from build123d import *

# Parameters (mm, degrees)
F1_DEPTH = 25.4
F2_R     = 6.35
F3_DEPTH = 12.7
F5_DEPTH = 25.4
F7_DEPTH = 12.7
F9_DEPTH = 12.7


with BuildPart() as f1:
    # F0 (on Front) → F1 (new body)
    with BuildSketch(Plane.XZ):
        Polygon((-56.1258053064, 50.8), (-68.8258053064, 50.8), (-68.8258053064, 0), (-11.6758053064, 0), (-11.6758053064, 12.7), (-56.1258053064, 12.7), align=None)
    extrude(amount=F1_DEPTH)

    # F2 (on face) → F3 (cut)
    with BuildSketch(Plane.XY.offset(12.7)):
        with Locations((-43.4258053064, -12.7)):
            Circle(F2_R)
        with Locations((-24.3758053064, -12.7)):
            Circle(F2_R)
    extrude(amount=-F3_DEPTH, mode=Mode.SUBTRACT)

    # F4 (on face) → F5 (cut)
    with BuildSketch(Plane.XY.offset(12.7)):
        with BuildLine():
            ThreePointArc((-24.3758053064, 0), (-15.3955491853, -3.7197438789), (-11.6758053064, -12.7))
            Line((-11.6758053064, -12.7), (-11.6758053064, 0))
            Line((-11.6758053064, 0), (-24.3758053064, 0))
        make_face()
        with BuildLine():
            Line((-11.6758053064, -25.4), (-11.6758053064, -12.7))
            ThreePointArc((-11.6758053064, -12.7), (-15.3955491853, -21.6802561211), (-24.3758053064, -25.4))
            Line((-24.3758053064, -25.4), (-11.6758053064, -25.4))
        make_face()
    extrude(amount=-F5_DEPTH, mode=Mode.SUBTRACT)

    # F6 (on face) → F7 (cut)
    with BuildSketch(Plane.YZ.offset(-56.1258053064)):
        with BuildLine():
            ThreePointArc((-19.040173462, 31.75), (-12.690173462, 38.1), (-6.340173462, 31.75))
            Line((-6.340173462, 31.75), (-6.340173462, 50.8))
            Line((-6.340173462, 50.8), (-19.040173462, 50.8))
            Line((-19.040173462, 50.8), (-19.040173462, 31.75))
        make_face()
        with BuildLine():
            ThreePointArc((-19.040173462, 31.75), (-12.690173462, 25.4), (-6.340173462, 31.75))
            ThreePointArc((-6.340173462, 31.75), (-12.690173462, 38.1), (-19.040173462, 31.75))
        make_face()
    extrude(amount=-F7_DEPTH, mode=Mode.SUBTRACT)

    # F8 (on face) → F9 (cut)
    with BuildSketch(Plane.YZ.offset(-56.1258053064)):
        with BuildLine():
            ThreePointArc((-25.4, 44.5000978606), (-22.682681328, 47.7661903137), (-19.040173462, 49.9532699015))
            Line((-19.040173462, 49.9532699015), (-19.040173462, 50.8))
            Line((-19.040173462, 50.8), (-25.4, 50.8))
            Line((-25.4, 50.8), (-25.4, 44.5000978606))
        make_face()
        with BuildLine():
            Line((-6.340173462, 50.8), (-6.340173462, 50.3012942354))
            ThreePointArc((-6.340173462, 50.3012942354), (-2.7361670375, 48.2166562079), (0, 45.0785089908))
            Line((0, 45.0785089908), (0, 50.8))
            Line((0, 50.8), (-6.340173462, 50.8))
        make_face()
    extrude(amount=-F9_DEPTH, mode=Mode.SUBTRACT)


solid = f1.part
Could you check a few things on this model? Use its own coordinates, in mm. A direction names the side the tool comes from. Round coordinates to 2 decimals unless told otherwise and drop trailing zeros. Write each loop counter-clockwise with the first axis right and the second up, starting at its lowest first coordinate (ties: lowest second). Pieces come first, ordered by that corner, then holes. Notation, with made-up numbers: (11.5, -16) - (51.5, -16) arc R18 ccw to (51.5, 4) - close; hole circle Ø6 at (48, 72.25). An arc over 180 degrees is marked (long way). Put each result on its own line as item: value. Start each with the question number.
(1) I want a section at B-B, the plane x = -45.5. Please give me the cut outline in (y, z).
(2) I want a section at D-D, the plane x = -52.5. Please give me the cut outline in (y, z), plus the area to 3 significant figures.
(3) For faces 5 (the flat face through (-62, -6.34, 41)), 6 (the flat face through (-34, -13, 12.7)), 7 (the cylindrical face through (-62.387, -2.781, 48.254)), which set-ups out of +Z, -Z, +X, -X, +Y, -Y let a thin tool reach every point of the face, with its end or its side?
(4) Thinking about a two-plate mould opening in X: for faces 1 (the cylindrical face through (-48.465, -16.564, 6.439)), 2 (the cylindrical face through (-62.4, -12.8, 25.4)), 3 (the flat face through (-56.126, -13, 23)), 4 (the cylindrical face through (-29.415, -16.564, 6.439)), which applies, released by +X, released by -X, zero draft, split by the parting line, or undercut?
(5) I want a section at A-A, the plane z = 33.5. Please give me the cut outline in (x, y).
(6) I need wall thicknesses on probe 1 along Y at (x, z) = (-64, 35.5); probe 2 along Z at (x, y) = (-52, -6); probe 3 along Y at (x, z) = (-65.5, 29). Which ranges of each line are inside material? Lowest first, please.
(7) Will these pins go through, and if not, where does the flat tip stop? pin 1 (12 mm diameter, centred on x = -48.5, z = 29.5, fed in from -Y); pin 2 (12.5 mm diameter, centred on x = -23, y = -15, fed in from +Z).
(8) I want a section at C-C, the plane y = -13.5. Please give me the cut outline in (x, z), plus the area to 3 significant figures.
Here are the results:
1. outline: (-25.4, 0) - (-18.7, 0) - (-18.7, 12.7) - (-25.4, 12.7) - close; (-6.7, 0) - (0, 0) - (0, 12.7) - (-6.7, 12.7) - close
2. outline: (-25.4, 0) - (0, 0) - (0, 12.7) - (-25.4, 12.7) - close
2. area: 323 mm^2
3. face 5: +Z, +X, -X
3. face 6: +Z, +X, +Y, -Y
3. face 7: +Z, +X, -X, +Y
4. face 1: undercut
4. face 2: zero draft
4. face 3: released by +X
4. face 4: undercut
5. outline: (-68.83, -25.4) - (-56.13, -25.4) - (-56.13, -19.04) - (-68.83, -19.04) - close; (-68.83, -6.34) - (-56.13, -6.34) - (-56.13, 0) - (-68.83, 0) - close
6. probe 1: y = -25.4 to -19.04, -6.34 to 0
6. probe 2: z = 0 to 12.7
6. probe 3: y = -25.4 to -18.41, -6.97 to 0
7. pin 1: passes through
7. pin 2: stops at z = 12.7
8. outline: (-68.83, 0) - (-49.73, 0) - (-49.73, 12.7) - (-56.13, 12.7) - (-56.13, 25.45) - (-68.83, 25.45) - close; (-37.13, 0) - (-30.68, 0) - (-30.68, 12.7) - (-37.13, 12.7) - close; (-18.08, 0) - (-11.7, 0) - (-11.7, 12.7) - (-18.08, 12.7) - close
8. area: 567 mm^2
